Design review of the part built by this model. Coordinates are the model's own, in mm. A direction names the side the tool comes from. Coordinates: 2 decimals unless noted, no trailing zeros. Write each loop counter-clockwise with the first axis right and the second up, starting at its lowest first coordinate (ties: lowest second). Pieces come first, ordered by that corner, then holes. Notation, with made-up numbers: M 53,9 L 77,9 A23 ccw 77,42 Z; hole C 39.5,39 d6. An arc over 180 degrees is marked long. Write item = value, one per line.
```python
from build123d import *

# Parameters (mm, degrees)
BOSS_EXTRUDE1_DEPTH = 22
CUT_EXTRUDE1_DEPTH  = 9
SKETCH3_R           = 5.1
CUT_EXTRUDE2_DEPTH  = 48.201694885
SHELL2_START        = 2
SHELL2_DEPTH        = 7
SHELL2_2_DEPTH      = 18
CUT_EXTRUDE4_DEPTH  = 47.957427527


# Read off the part's stored shape, not the designer's step: Shell2
with BuildPart() as part:
    # Sketch1 → Boss-Extrude1 (new body)
    with BuildSketch(Plane.XY):
        Polygon((0, 0), (3, 0), (0, -3), (10, -3), (7, 0), (33, 0), (30, -3), (40, -3), (37, 0), (40, 0), (40, 11), (0, 11), align=None)
    extrude(amount=BOSS_EXTRUDE1_DEPTH)

    # Sketch2 → Cut-Extrude1 (cut)
    with BuildSketch(Plane(origin=(0, 0, 0), x_dir=(-1, 0, 0), z_dir=(0, -1, 0))):
        Polygon((-14.803847577, -20), (-25.196152423, -20), (-30.392304845, -11), (-25.196152423, -2), (-14.803847577, -2), (-9.607695155, -11), align=None)
    extrude(amount=-CUT_EXTRUDE1_DEPTH, mode=Mode.SUBTRACT)

    # Sketch3 → Cut-Extrude2 (cut, through all)
    with BuildSketch(Plane(origin=(0, 9, 0), x_dir=(-1, 0, 0), z_dir=(0, -1, 0))):
        with Locations(Location((-20, -11, 0), (0, 0, 180))):
            Circle(SKETCH3_R)
    extrude(amount=-CUT_EXTRUDE2_DEPTH, mode=Mode.SUBTRACT)

    # Shell2 outline → Shell2 (cut)
    with BuildSketch(Plane(origin=(0, 0, 0), x_dir=(1, 0, 0), z_dir=(0, 1, 0)).offset(SHELL2_START)):
        Polygon((2, -2), (2, -20), (12.494446501, -20), (7.298294078, -11), (12.494446501, -2), align=None)
        Polygon((32.701705922, -11), (27.505553499, -20), (38, -20), (38, -2), (27.505553499, -2), align=None)
    extrude(amount=SHELL2_DEPTH, mode=Mode.SUBTRACT)

    # Shell2 2 outline → Shell2 2 (cut)
    with BuildSketch(Plane.XY.offset(SHELL2_START)):
        Polygon((5.171572875, -1), (5, -0.828427125), (4.828427125, -1), align=None)
        Polygon((34.828427125, -1), (35.171572875, -1), (35, -0.828427125), align=None)
    extrude(amount=SHELL2_2_DEPTH, mode=Mode.SUBTRACT)

    # Sketch6 → Cut-Extrude4 (cut, through all)
    with BuildSketch(Plane.XY.offset(22)):
        Polygon((31.707106781, -2.292893219), (34, 0), (33, 0), (30, -3), (40, -3), (37, 0), (36, 0), (38.292893219, -2.292893219), align=None)
        Polygon((1.707106781, -2.292893219), (4, 0), (3, 0), (0, -3), (10, -3), (7, 0), (6, 0), (8.292893219, -2.292893219), align=None)
    extrude(amount=-CUT_EXTRUDE4_DEPTH, mode=Mode.SUBTRACT)


solid = part.part
```
Q1. For P1, Ø1.5, axis at x = 17.5, z = 8, coming from the -Y side, flat-tipped, find the tip position at first contact; note if it passes through.
Check result:
P1 = through
Q2. Consider section D-D, the plane x = 20. State the section outline as (y, z) points, and give its area (3 significant figures).
Check result:
outline = M 0,0 L 11,0 L 11,5.9 L 9,5.9 L 9,2 L 0,2 Z; M 0,20 L 9,20 L 9,16.1 L 11,16.1 L 11,22 L 0,22 Z
area = 59.6 mm²
Q3. Consider section C-C, the plane y = 8. State the section outline as (x, z) points.
Check result:
outline = M 0,0 L 40,0 L 40,22 L 0,22 Z; hole M 2,2 L 12.49,2 L 7.3,11 L 12.49,20 L 2,20 Z; hole M 9.61,11 L 14.8,2 L 25.2,2 L 30.39,11 L 25.2,20 L 14.8,20 Z; hole M 27.51,2 L 38,2 L 38,20 L 27.51,20 L 32.7,11 Z
Q4. Wall thickness on line 1 (Z direction, x = 20, y = 9.9); line 2 (Z direction, x = 17, y = 1.75); line 3 (X direction, y = 8, z = 12.5): over which ranges is each line inside the solid? List them lowest first.
Check result:
line_1 = 0 to 5.9, 16.1 to 22
line_2 = 0 to 2, 20 to 22
line_3 = 0 to 2, 8.16 to 10.47, 29.53 to 31.84, 38 to 40
Q5. Machinability: for faces 5 (the flat face through (15, 9, 13)), 6 (the flat face through (9.93, 5.45, 15.56)), 7 (the flat face through (38, 0, 11)), which of the approach directions +Z, -Z, +X, -X, +Y, -Y give a long, thin tool a straight path to every point of the face, cutting with its end or side? Answer none if there is none.
Check result:
face_5 = -Y
face_6 = none
face_7 = +Z, -Z, +X
Q6. The part is to be moulded in two halves that separate along Y. For faces 1 (the flat face through (12.24, 4.44, 6.44)), 2 (the flat face through (25, 11, 8)), 3 (the flat face through (30.14, 5.45, 15.44)), 4 (the flat face through (35, -2.293, 11)), say which applies: +Y half, -Y half, draft (parallel to the pull), parting line (faces both ways), or undercut.
Check result:
face_1 = draft
face_2 = +Y half
face_3 = undercut
face_4 = -Y half
Q7. Consider section A-A, the plane x = 33.5. State the section outline as (y, z) points, and give its area (3 significant figures).
Check result:
outline = M -2.29,0 L -0.5,0 L -0.5,22 L -2.29,22 Z; M 0,0 L 11,0 L 11,22 L 0,22 Z; hole M 2,2 L 9,2 L 9,20 L 2,20 Z
area = 155 mm²
Q8. Consider section B-B, the plane z = 12.75. State how many separate pieces and enclosed holes the cut face has, and give its area (3 significant figures).
Check result:
separate_pieces = 2
enclosed_holes = 4
area = 183 mm²
